The model under review builds one solid part; all positions refer to its coordinate system, in mm. Face numbers are marked on the shaded views. A direction names the side the tool comes from. Round coordinates to 2 decimals unless told otherwise and drop trailing zeros. Order: outer loops, then holes, each group sorted by start corner. A loop starts at its lowest first (then second) coordinate and runs counter-clockwise, first axis right, second up. Notation, with made-up numbers: M 9,42.5 L 20,42.5 A14 ccw 20,54.5 Z; hole C 66.25,24 d5. An arc over 180 degrees is marked long. Answer as a JSON object with one key per item and string values. Group by question number.
1. Mouldability with a two-part tool opening along Z and no side actions: class the marked faces 3, 4 and 5 as released by +Z, released by -Z, zero draft, split by the parting line, or undercut.
2. Machinability: for the marked faces 1 and 2, which of the approach directions +Z, -Z, +X, -X, +Y, -Y give a long, thin tool a straight path to every point of the face, cutting with its end or side? Answer none if there is none.
3. Clearance check with flat-ended pins moving along their axes: P1, Ø2.5, axis at x = 0.5, z = 16.5, coming from the +Y side (3 decimals); P2, Ø1.9, axis at x = -0.5, z = 10, coming from the +Y side. State where each tip first meets the part, or that it passes through.
4. Add section A-A on x = 0. State the section outline as (y, z) points (3 decimals), and give its area (3 significant figures).
5. Add section C-C on y = 13.25. State the section outline as (x, z) points (3 decimals).
6. Add section B-B on z = 4.75. State the section outline as (x, y) points (3 decimals), and give its area (3 significant figures).
7. To check wall thickness, follow probe 1 along Y at (x, z) = (0.75, 2.5); probe 2 along Z at (x, y) = (-2, -1.25); probe 3 along Z at (x, y) = (-0.25, 14.75). State the ranges of each line that lie inside material, in increasing order. Write a range as [from, to].
8. Add section D-D on x = -2.5. State the section outline as (y, z) points, and give its area (3 significant figures).
```python
from build123d import *

# Parameters (mm, degrees)
F0_W     = 6.35
F0_H     = 25.4
F1_DEPTH = 19.05
F2_SIZE  = 10.16
F3_R     = 1.27
F4_R     = 1.27
F5_R     = 1.905
F6_DEPTH = 3.175


with BuildPart() as f1:
    # F0 (on Top) → F1 (new body)
    with BuildSketch(Plane.XY):
        Rectangle(F0_W, F0_H)
    extrude(amount=F1_DEPTH)

    # F2
    f2_edges = [f1.edges().sort_by_distance(p)[0] for p in [
        (0, -12.7, 19.05),
    ]]
    chamfer(f2_edges, length=F2_SIZE)

    # F3
    f3_edges = [f1.edges().sort_by_distance(p)[0] for p in [
        (0, 12.7, 19.05),
        (0, -2.54, 19.05),
        (0, -12.7, 8.89),
    ]]
    fillet(f3_edges, radius=F3_R)

    # F4
    f4_edges = [f1.edges().sort_by_distance(p)[0] for p in [
        (3.175, -12.7, 4.181974),
        (3.175, -7.62, 13.97),
        (-3.175, -12.7, 4.181974),
        (-3.175, -7.62, 13.97),
        (-3.175, -12.603327, 8.849957),
        (3.175, -12.603327, 8.849957),
        (3.175, -2.499957, 18.953327),
        (3.175, 4.708026, 19.05),
        (-3.175, -2.499957, 18.953327),
        (-3.175, 4.708026, 19.05),
        (-3.175, 12.328026, 18.678026),
        (3.175, 12.328026, 18.678026),
        (3.175, 12.7, 8.89),
        (-3.175, 12.7, 8.89),
    ]]
    fillet(f4_edges, radius=F4_R)

    # F5 (on face) → F6 (join)
    with BuildSketch(Plane(origin=(0, 12.7, 0), x_dir=(-1, 0, 0), z_dir=(0, 1, 0))):
        with Locations((0, 14.4283687696)):
            Circle(F5_R)
        with Locations((0, 5.5899028666)):
            Circle(F5_R)
    extrude(amount=F6_DEPTH)


solid = f1.part
```
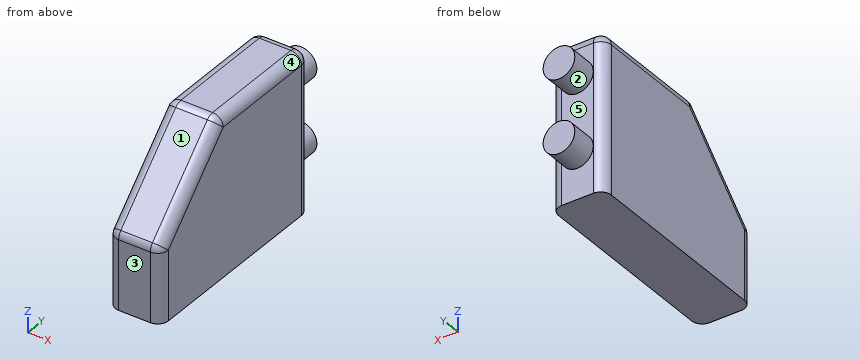
Recorded:
{
 "1": {"face 3": "zero draft", "face 4": "released by +Z", "face 5": "undercut"},
 "2": {"face 1": "+Z, +X, -X, -Y", "face 2": "+Y"},
 "3": {"P1": "stops at y = 15.875", "P2": "stops at y = 12.7"},
 "4": {"outline": "M -12.7,0 L 12.7,0 L 12.7,3.685 L 15.875,3.685 L 15.875,7.495 L 12.7,7.495 L 12.7,12.523 L 15.875,12.523 L 15.875,16.333 L 12.7,16.333 L 12.7,17.78 A1.27 ccw 11.43,19.05 L -2.014,19.05 A1.27 ccw -2.912,18.678 L -12.328,9.262 A1.27 ccw -12.7,8.364 Z", "area": "456 mm²"},
 "5": {"outline": "C 0,5.59 d3.81; C 0,14.428 d3.81"},
 "6": {"outline": "M -3.175,-11.43 A1.27 ccw -1.905,-12.7 L 1.905,-12.7 A1.27 ccw 3.175,-11.43 L 3.175,11.43 A1.27 ccw 1.905,12.7 L 1.71,12.7 L 1.71,15.875 L -1.71,15.875 L -1.71,12.7 L -1.905,12.7 A1.27 ccw -3.175,11.43 Z", "area": "171 mm²"},
 "7": {"probe 1": "y = [-12.7, 12.7]", "probe 2": "z = [0, 19.05]", "probe 3": "z = [3.7, 7.48], [12.54, 16.32]"},
 "8": {"outline": "M -12.55,0 L 12.55,0 L 12.55,17.78 A1.12 ccw 11.43,18.9 L -2.01,18.9 A1.12 ccw -2.81,18.57 L -12.22,9.16 A1.12 ccw -12.55,8.36 Z", "area": "423 mm²"}
}
